```python
from build123d import *

# Parameters (mm, degrees)
F0_W      = 50.8
F0_H      = 50.8
F1_DEPTH  = 135.89
F6_DEPTH  = 50.8
F11_W     = 12.7
F11_H     = 15.1711734065
F12_DEPTH = 27.7114
F13_DEPTH = 36.9062
F14_DEPTH = 15.1721734065
F17_DEPTH = 5.8166
F18_DEPTH = 25.654
F20_DEPTH = 50.8
F23_DEPTH = 9.906
F24_DEPTH = 28.194
F26_DEPTH = 3.556
F27_DEPTH = 33.528
F29_DEPTH = 12.7
F31_DEPTH = 12.7


with BuildPart() as f1:
    # F0 (on Top) → F1 (new body)
    with BuildSketch(Plane.XY):
        with Locations((4.8314797107, 4.7515430488)):
            Rectangle(F0_W, F0_H)
    extrude(amount=F1_DEPTH)

    # F5 (on face) + F3 (on face) → F6 (cut)
    with BuildSketch(Plane(origin=(-20.5685202893, 0, 0), x_dir=(0, -1, 0), z_dir=(-1, 0, 0))):
        Polygon((-4.7515430488, 120.7188265935), (-4.7515430488, 135.89), (-30.1515430488, 120.7188265935), align=None)
    with BuildSketch(Plane(origin=(-20.5685202893, 0, 0), x_dir=(0, -1, 0), z_dir=(-1, 0, 0))):
        Polygon((-30.1515430488, 135.89), (-30.1515430488, 120.7188265935), (-4.7515430488, 135.89), align=None)
    extrude(amount=-F6_DEPTH, mode=Mode.SUBTRACT)

    # F11 (on face) → F12 (join)
    with BuildSketch(Plane(origin=(0, 30.1515430488, 0), x_dir=(-1, 0, 0), z_dir=(0, 1, 0))):
        with Locations((-4.8314797107, 128.3044132968)):
            Rectangle(F11_W, F11_H)
    extrude(amount=-F12_DEPTH)

    # F2 (on face) → F13 (join)
    with BuildSketch(Plane(origin=(0, 30.1515430488, 0), x_dir=(-1, 0, 0), z_dir=(0, 1, 0))):
        Polygon((7.8685202893, 135.89), (-17.5314797107, 135.89), (-11.1814797107, 120.7188265935), (1.5185202893, 120.7188265935), align=None)
    extrude(amount=-F13_DEPTH)

    # F4 (on face) → F14 (cut, through all)
    with BuildSketch(Plane.XY.offset(135.89)):
        Polygon((17.5314797107, 4.7515430488), (17.5314797107, 30.1515430488), (11.1814797107, 4.7515430488), align=None)
    extrude(amount=-F14_DEPTH, mode=Mode.SUBTRACT)

    # F16 (on 3pt) → F17 (cut)
    with BuildSketch(Plane(origin=(-37.880335568, 9.470083892, 15.8550775482), x_dir=(-0.2072908126, -0.9744242912, 0.0867630094), z_dir=(-0.8988641792, 0.2247160448, 0.3762258452))):
        Polygon((4.8423883579, 129.6698123278), (-21.2242852978, 132.1215514099), (-21.2242852978, 115.6750623459), (3.5260916978, 115.6750623459), align=None)
    extrude(amount=-F17_DEPTH, mode=Mode.SUBTRACT)

    # F18 (add): a face of the model
    f18_faces = [f1.faces().sort_by_distance(p)[0] for p in [
        (30.2314797107, 4.0006963035, 64.3764433841),
    ]]
    extrude(f18_faces, amount=-F18_DEPTH)

    # F19 (on face) → F20 (join)
    with BuildSketch(Plane.YZ.offset(30.2314797107)):
        Polygon((30.1515430488, 120.7188265935), (4.7515430488, 135.89), (4.7515430488, 120.7188265935), align=None)
    extrude(amount=-F20_DEPTH)

    # F22 (on 3pt) → F23 (cut)
    with BuildSketch(Plane(origin=(45.6875894624, 11.4218973656, 19.1228578906), x_dir=(-0.2072908126, 0.9744242912, -0.0867630094), z_dir=(0.8988641792, 0.2247160448, 0.3762258452))):
        Polygon((19.221242587, 111.9441875016), (19.221242587, 128.4180545008), (-6.8454310687, 125.9389374835), (-5.5291344086, 111.9441875016), align=None)
    extrude(amount=-F23_DEPTH, mode=Mode.SUBTRACT)

    # F24 (add): a face of the model
    f24_faces = [f1.faces().sort_by_distance(p)[0] for p in [
        (-20.5685202893, 4.2653508293, 66.1393526656),
    ]]
    extrude(f24_faces, amount=-F24_DEPTH)

    # F25 (on face) → F26 (cut)
    with BuildSketch(Plane.XY.offset(135.89)):
        Polygon((-7.8685202893, 4.7515430488), (-1.5185202893, 4.7515430488), (-7.8685202893, 29.8561221751), align=None)
    extrude(amount=-F26_DEPTH, mode=Mode.SUBTRACT)

    # F27 (add): a face of the model
    f27_faces = [f1.faces().sort_by_distance(p)[0] for p in [
        (-20.5685202893, 4.2653508293, 66.1393526656),
    ]]
    extrude(f27_faces, amount=-F27_DEPTH)

    # F28 (on face) → F29 (cut)
    with BuildSketch(Plane.YZ.offset(30.2314797107)):
        Polygon((-20.6484569512, 135.89), (-20.6484569512, 120.7188265935), (4.7515430488, 135.89), align=None)
    extrude(amount=-F29_DEPTH, mode=Mode.SUBTRACT)

    # F30 (on face) → F31 (cut)
    with BuildSketch(Plane(origin=(-20.5685202893, 0, 0), x_dir=(0, -1, 0), z_dir=(-1, 0, 0))):
        Polygon((-4.7515430488, 135.89), (20.6484569512, 120.7188265935), (20.6484569512, 135.89), align=None)
    extrude(amount=-F31_DEPTH, mode=Mode.SUBTRACT)


solid = f1.part
```
Geometry: final body of the model. Coordinates: model frame, mm. A direction names the side the tool comes from. Coordinates: 2 decimals unless noted, no trailing zeros. Order: outer loops, then holes, each group sorted by start corner. A loop starts at its lowest first (then second) coordinate and runs counter-clockwise, first axis right, second up. Notation, with made-up numbers: (75, -36) - (93, -36) arc R20 ccw to (93, -18) - close; hole circle Ø10 at (-22, -34). An arc over 180 degrees is marked (long way). Return JSON: item names as keys, results as strings. Group by question number.
1. Pin query (flat end, axial travel): pin 1 (8 mm diameter, centred on x = 24, y = 8.5, fed in from +Z); pin 2 (2 mm diameter, centred on x = -14.5, y = 9.5, fed in from +Z). Return the tip coordinate at first contact, or that it passes through.
2. Set-up query: faces 4 (the face through (30.231, 4, 69)), 5 (the face through (17.531, -11, 130)), 6 (the face through (13.043, 20.452, 130.96)), 7 (the face through (-10.91, 17.63, 128.2)), 8 (the face through (-14.31, -7.77, 128.41)). Return all of +Z, -Z, +X, -X, +Y, -Y with unobstructed straight access to the full face (end or side cutting, diameter ignored); none if empty.
3. Cut plane A-A (x = 14.5). Output: boundary loops of the cut face in (y, z), plus the area to 3 significant figures.
4. Cut plane C-C (x = -4). Output: boundary loops of the cut face in (y, z).
5. Material intervals for line 1 along Z through (x, y) = (-16, -4.5); line 2 along Z through (x, y) = (-11, 21), sorted ascending. Write a range as [from, to].
6. Cut plane B-B (y = 25.5). Output: boundary loops of the cut face in (x, z).
7. Pull-direction query (Y, two-part tool) for faces 1 (the face through (5, 5, 135.89)), 2 (the face through (4, -20.648, 67)), 3 (the face through (-3.905, 22.918, 130.74)); classes: pulls with the +Y half, pulls with the -Y half, needs draft (parallel to the pull), parting line crosses it, or undercut.
8. Cut plane D-D (y = -5.5). Output: boundary loops of the cut face in (x, z), plus the area to 3 significant figures.
Resolved:
{
 "1": {"pin 1": "stops at z = 135.89", "pin 2": "stops at z = 133.65"},
 "2": {"face 4": "+Z, -Z, +X, +Y, -Y", "face 5": "+Z, +X, -Y", "face 6": "+X", "face 7": "-X", "face 8": "+Z, -X, -Y"},
 "3": {"outline": "(-20.65, 0) - (30.15, 0) - (30.15, 120.72) - (4.75, 135.89) - (-20.65, 135.89) - close; (18.03, 135.89) - (30.15, 128.65) - (30.15, 135.89) - close", "area": "6,750 mm²"},
 "4": {"outline": "(-20.65, 0) - (30.15, 0) - (30.15, 120.72) - (4.75, 135.89) - (-20.65, 135.89) - close; (14.68, 135.89) - (30.15, 126.65) - (30.15, 135.89) - close"},
 "5": {"line 1": "z = [0, 130.36]", "line 2": "z = [0, 126.18]"},
 "6": {"outline": "(-20.57, 0) - (30.23, 0) - (30.23, 123.5) - (11.18, 123.5) - (16.37, 135.89) - (-6.71, 135.89) - (-1.52, 123.5) - (-20.57, 123.5) - close"},
 "7": {"face 1": "needs draft", "face 2": "pulls with the -Y half", "face 3": "undercut"},
 "8": {"outline": "(-20.57, 0) - (30.23, 0) - (30.23, 129.77) - (17.53, 129.77) - (17.53, 135.89) - (-7.87, 135.89) - (-7.87, 129.77) - (-20.57, 129.77) - close", "area": "6,750 mm²"}
}
